```python
from build123d import *


with BuildPart() as part:
    # Esquisse1 → Révolution3 (revolve)
    with BuildSketch(Plane(origin=(0, 0, 0), x_dir=(0, 0, -1), z_dir=(1, 0, 0))):
        with BuildLine():
            Line((31.25, 0), (28.273835099, 0))
            ThreePointArc((28.273835099, 0), (20.499905423, 38.067161735), (19.497117554, 76.90705362))
            ThreePointArc((19.497117554, 76.90705362), (19.093027806, 78.027273194), (18, 78.5))
            Line((18, 78.5), (17.628058133, 78.5))
            ThreePointArc((17.628058133, 78.5), (16.912594573, 78.318374717), (16.370392708, 77.817482526))
            Line((16.370392708, 77.817482526), (4.789029066, 60))
            Line((4.789029066, 60), (3, 60))
            Line((3, 60), (15.112727284, 78.634965052))
            ThreePointArc((15.112727284, 78.634965052), (16.197131013, 79.636749434), (17.628058133, 80))
            Line((17.628058133, 80), (18, 80))
            ThreePointArc((18, 80), (20.186055613, 79.054546388), (20.994235108, 76.814107239))
            ThreePointArc((20.994235108, 76.814107239), (21.857795657, 39.426427354), (29.041387811, 2.725196477))
            ThreePointArc((29.041387811, 2.725196477), (29.400726908, 2.201625551), (30.002888214, 2))
            Line((30.002888214, 2), (31.25, 2))
            Line((31.25, 2), (31.25, 0))
        make_face()
    revolve(axis=Axis((0, 0, 0), (0, 1, 0)))


solid = part.part
```
Can you work these out from the model? Positions are in its coordinate system, mm. A direction names the side the tool comes from. Give positions to 0.01 mm unless a question says otherwise; leave off trailing zeros. Order: outer loops, then holes, each group sorted by start corner. A loop starts at its lowest first (then second) coordinate and runs counter-clockwise, first axis right, second up. Notation, with made-up numbers: (74.25, 57) - (81.25, 57) arc R30 ccw to (81.25, 81) - close; hole circle Ø4 at (-13, 47.25). An arc over 180 degrees is marked (long way). Use a Markdown table: item, result. Add a question column.
Q1. If we mould it in two halves opening along X, with no side actions, what happens to faces 1 (the conical face through (7.737, 64.825, 1.718)), 2 (the flat face through (28, 0, 7)), 3 (the cylindrical face through (-1.37, 0.99, 31.22))? For each: released by +X, released by -X, zero draft, split by the parting line, or undercut.
Q2. On a 3-axis mill with a long thin cutter (end or side, diameter ignored), from which of +Z, -Z, +X, -X, +Y, -Y can I reach the whole of each face in a straight line? I mean faces 4 (the flat face through (13.25, 80, 11.92)), 5 (the flat face through (-12, 2, -28)), 6 (the flat face through (13.25, 78.5, -11.92)). Say none if no direction works.
Q3. Please list where these lines run through material, in increasing order: line 1 along Z through (x, y) = (-0.5, 65); line 2 along Z through (x, y) = (-4.5, 69); line 3 along Z through (x, y) = (-16.5, 69.5).
Q4. If we section it at C-C on y = 8.5: Write out the boundary of the cut face in (x, z).
Q5. I'm going to push flat-ended pins straight in: pin 1 (4 mm diameter, centred on y = 24.5, z = 14.5, fed in from +X); pin 2 (18 mm diameter, centred on x = 3, z = 5.5, fed in from -Y); pin 3 (5 mm diameter, centred on y = 25.5, z = 9, fed in from +X). Where does each tip first touch, or does it pass through?
Answers follow:
| question | item | result |
|---|---|---|
| 1 | face 1 | undercut |
| 1 | face 2 | zero draft |
| 1 | face 3 | split by the parting line |
| 2 | face 4 | +Z, -Z, +X, -X, +Y |
| 2 | face 5 | +Y |
| 2 | face 6 | -Y |
| 3 | line 1 | z = -20.57 to -19.07, -8.02 to -6.23, 6.23 to 8.02, 19.07 to 20.57 |
| 3 | line 2 | z = -20.15 to -18.61, -9.64 to -7.62, 7.62 to 9.64, 18.61 to 20.15 |
| 3 | line 3 | z = -12.44 to -9.74, 9.74 to 12.44 |
| 4 | outline | circle Ø54.95 at (0, 0); hole circle Ø51.85 at (0, 0) |
| 5 | pin 1 | stops at x = 20.56 |
| 5 | pin 2 | stops at y = 60 |
| 5 | pin 3 | stops at x = 23.05 |
